Drawing for the job (mm, zero at the part's lowest x, y, z). Coordinates: 2 decimals unless noted, no trailing zeros. Loops run counter-clockwise (first coordinate to the right, second up) from the corner with the lowest first, then second, coordinate; pieces in that order, holes last. Notation, with made-up numbers: (-18.5, -30.5) -> (9.5, -30.5) arc R25 cw to (9.5, -5.5) -> close; hole circle Ø6 at (43, 69). An arc over 180 degrees is marked (long way). Write item = value, one per line. Start each with the question number.
(1) Band-saw the part on D-D (z = 49). Write the cut outline in (x, y) (1 decimal).
(2) Flat gauge pins, fed straight in: P1, Ø3, axis at x = 42, z = 52.5, coming from the -Y side; P2, Ø1.1, axis at x = 52.5, z = 2.5, coming from the +Y side. Where does each tip first touch, or does it go through?
(3) Band-saw the part on A-A (x = 16.5). Write the cut outline in (y, z) (1 decimal), and give its area (3 significant figures).
(4) Band-saw the part on C-C (x = 2.5). Write the cut outline in (y, z) (1 decimal).
(5) Drill centre lines: line 1 (X direction, y = 1.95, z = 2.5); line 2 (Z direction, x = 2.5, y = 2.45); line 3 (Z direction, x = 16.5, y = 0.35). Where is each one in solid material? Low to high. Write a range as from..to.
(6) Band-saw the part on B-B (z = 2.5). Write the cut outline in (x, y) (1 decimal), and give its area (3 significant figures).
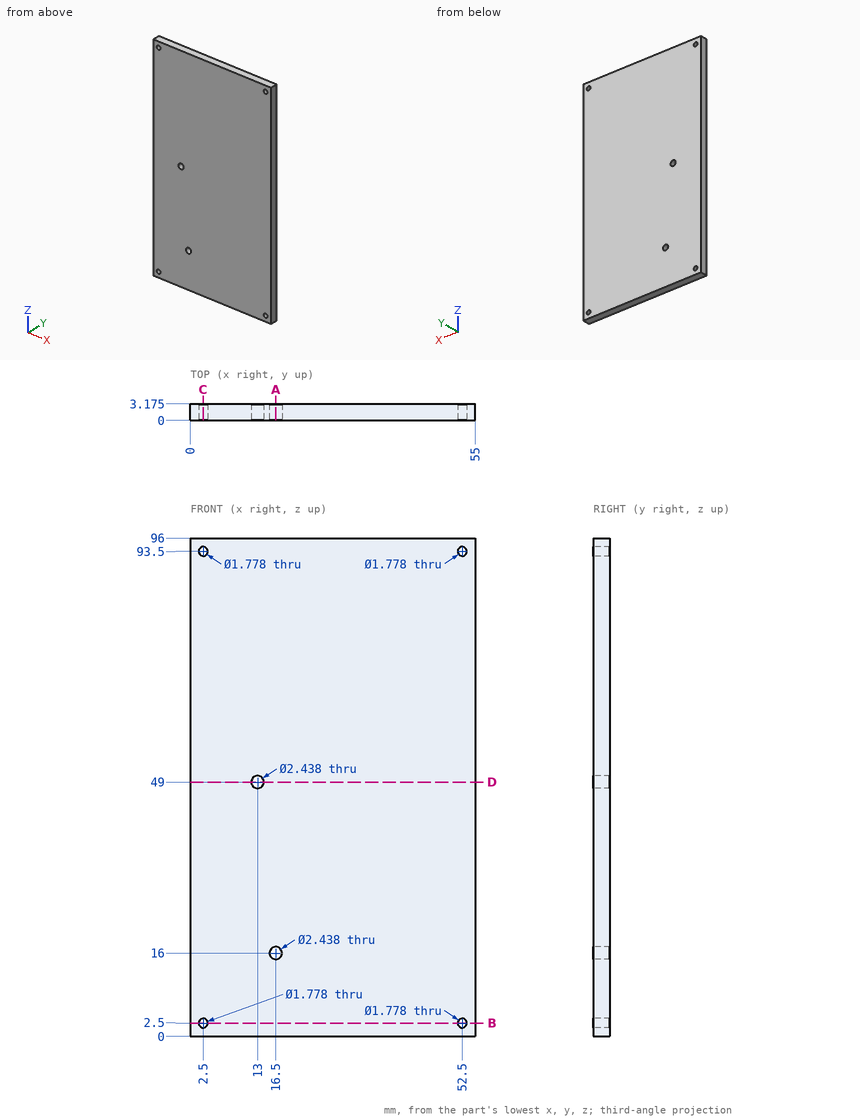
Findings below:
q1.outline = (0, 0) -> (11.8, 0) -> (11.8, 3.2) -> (0, 3.2) -> close; (14.2, 0) -> (55, 0) -> (55, 3.2) -> (14.2, 3.2) -> close
q2.P1 = 0
q2.P2 = through
q3.outline = (0, 0) -> (3.2, 0) -> (3.2, 14.8) -> (0, 14.8) -> close; (0, 17.2) -> (3.2, 17.2) -> (3.2, 96) -> (0, 96) -> close
q3.area = 297 mm²
q4.outline = (0, 0) -> (3.2, 0) -> (3.2, 1.6) -> (0, 1.6) -> close; (0, 3.4) -> (3.2, 3.4) -> (3.2, 92.6) -> (0, 92.6) -> close; (0, 94.4) -> (3.2, 94.4) -> (3.2, 96) -> (0, 96) -> close
q5.line_1 = 0..1.61, 3.39..51.61, 53.39..55
q5.line_2 = 0..1.61, 3.39..92.61, 94.39..96
q5.line_3 = 0..14.78, 17.22..96
q6.outline = (0, 0) -> (1.6, 0) -> (1.6, 3.2) -> (0, 3.2) -> close; (3.4, 0) -> (51.6, 0) -> (51.6, 3.2) -> (3.4, 3.2) -> close; (53.4, 0) -> (55, 0) -> (55, 3.2) -> (53.4, 3.2) -> close
q6.area = 163 mm²
